Verification items for the finished model (mm, model axes). Face numbers are marked on the shaded views. Coordinates: 2 decimals unless noted, no trailing zeros. Loops run counter-clockwise (first coordinate to the right, second up) from the corner with the lowest first, then second, coordinate; pieces in that order, holes last. Notation, with made-up numbers: (-34, 0.5) -> (17, 0.5) arc R25 cw to (17, 29.5) -> close; hole circle Ø7 at (-34.75, 56). An arc over 180 degrees is marked (long way). Use CSV: the item, a comma, the result in double quotes. Start each with the question number.
```python
from build123d import *

# Parameters (mm, degrees)
SKETCH2_W           = 31.75
SKETCH2_H           = 23.368
BOSS_EXTRUDE1_DEPTH = 2.54
SKETCH3_W           = 12.7
SKETCH3_H           = 1.778
BOSS_EXTRUDE2_DEPTH = 6.35
SKETCH4_W           = 2.54
SKETCH4_H           = 6.35
CUT_EXTRUDE1_DEPTH  = 24.368


with BuildPart() as part:
    # Sketch2 → Boss-Extrude1 (new body)
    with BuildSketch(Plane.XY):
        Rectangle(SKETCH2_W, SKETCH2_H)
    extrude(amount=BOSS_EXTRUDE1_DEPTH)

    # Sketch3 → Boss-Extrude2 (add)
    with BuildSketch(Plane.XY.offset(2.54)):
        with Locations((9.525, 10.795)):
            Rectangle(SKETCH3_W, SKETCH3_H)
        with Locations((9.525, -10.795)):
            Rectangle(SKETCH3_W, SKETCH3_H)
    extrude(amount=BOSS_EXTRUDE2_DEPTH)

    # Sketch4 → Cut-Extrude1 (cut, through all)
    with BuildSketch(Plane(origin=(0, 11.684, 0), x_dir=(1, 0, 0), z_dir=(0, 1, 0))):
        with Locations((14.605, -5.715)):
            Rectangle(SKETCH4_W, SKETCH4_H)
    extrude(amount=-CUT_EXTRUDE1_DEPTH, mode=Mode.SUBTRACT)


solid = part.part
```
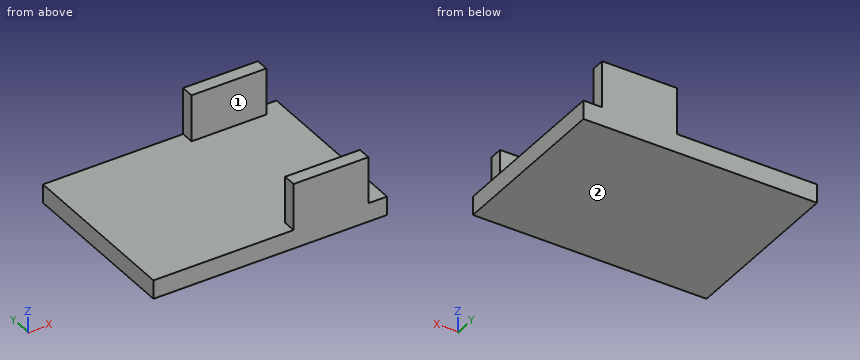
1. Cross-section at C-C, the plane x = -11. Record the boundary of the cut face in (y, z).
2. Cross-section at B-B, the plane y = -4.5. Record the boundary of the cut face in (x, z) (3 decimals).
3. Depth check by flat-ended pin: pin 1 (7 mm diameter, centred on x = 2, y = -5.5, fed in from +Z); pin 2 (0.9 mm diameter, centred on y = 10.5, z = 5, fed in from -X) (3 decimals); pin 3 (1.4 mm diameter, centred on y = 10.5, z = 5.5, fed in from +X) (3 decimals); pin 4 (4 mm diameter, centred on y = 6.5, z = 6.5, fed in from -X). Enter the tip coordinate at first touch or a pass-through.
4. Scan lines: line 1 (Y direction, x = 11, z = 3); line 2 (X direction, y = -10.5, z = 5.25) (3 decimals); line 3 (Z direction, x = 2, y = -1.75). Record each from-to range of solid material in increasing order.
5. Cross-section at A-A, the plane z = 3. Record the boundary of the cut face in (x, y) (3 decimals), plus the area to 3 significant figures.
6. Release check for a two-part mould opening along Z. For the marked faces 1 and 2 record: released by +Z, released by -Z, zero draft, split by the parting line, or undercut.
Solution:
1,outline,"(-11.68, 0) -> (11.68, 0) -> (11.68, 2.54) -> (-11.68, 2.54) -> close"
2,outline,"(-15.875, 0) -> (15.875, 0) -> (15.875, 2.54) -> (-15.875, 2.54) -> close"
3,pin 1,"stops at z = 2.54"
3,pin 2,"stops at x = 3.175"
3,pin 3,"stops at x = 13.335"
3,pin 4,"passes through"
4,line 1,"y = -11.68 to -9.91, 9.91 to 11.68"
4,line 2,"x = 3.175 to 13.335"
4,line 3,"z = 0 to 2.54"
5,outline,"(3.175, -11.684) -> (13.335, -11.684) -> (13.335, -9.906) -> (3.175, -9.906) -> close; (3.175, 9.906) -> (13.335, 9.906) -> (13.335, 11.684) -> (3.175, 11.684) -> close"
5,area,"36.1 mm2"
6,face 1,"zero draft"
6,face 2,"released by -Z"
